Part print with two shaded views. Sizes in mm from the minimum x, y, z corner. Give positions to 0.01 mm unless a question says otherwise; leave off trailing zeros. Order: outer loops, then holes, each group sorted by start corner. A loop starts at its lowest first (then second) coordinate and runs counter-clockwise, first axis right, second up. Notation, with made-up numbers: M 3.25,5 L 27.25,5 A22 cw 27.25,16 Z; hole C 59,-27.75 d6. An arc over 180 degrees is marked long. Write each question's results on one line, items separated by ' | '. Start each with the question number.
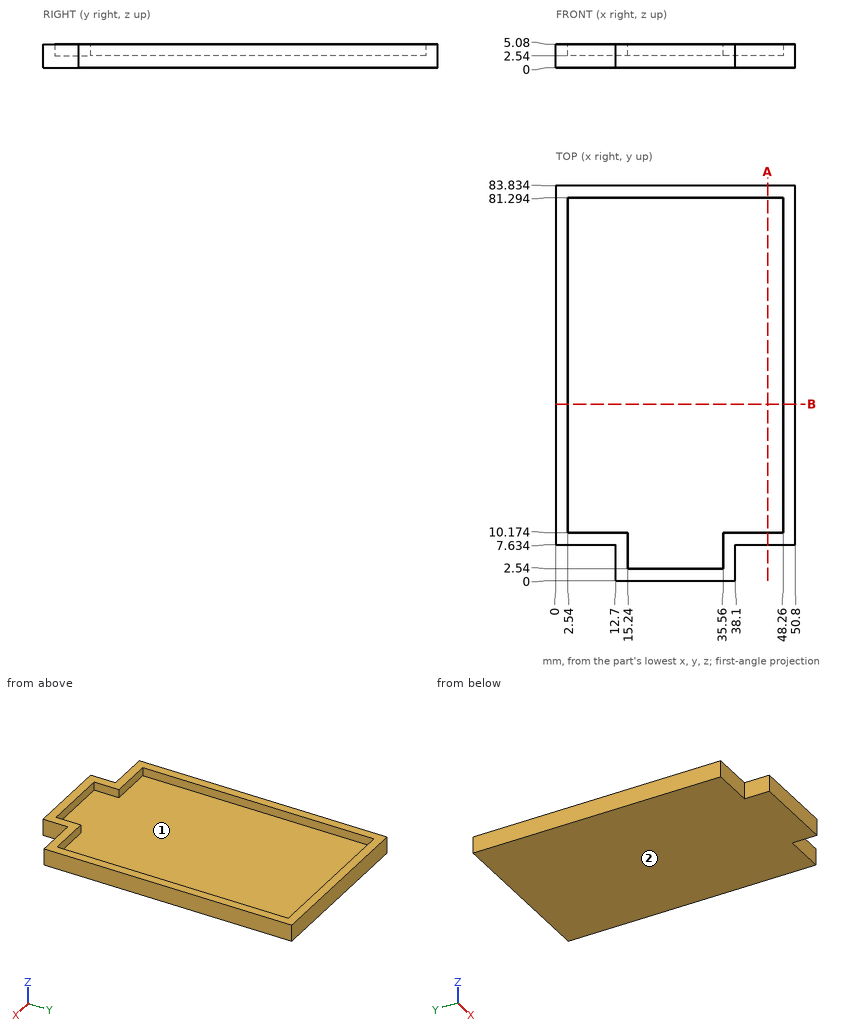
(1) Pull direction Y, two halves, no side cores. Call the marked faces 1 and 2: +Y half, -Y half, draft (parallel to the pull), parting line (faces both ways), or undercut.
(2) Drop flat-ended pins along their axis: P1, Ø4, axis at x = 45.5, y = 31.5, coming from the +Z side; P2, Ø1.3, axis at y = 6.5, z = 3.5, coming from the -X side; P3, Ø2.5, axis at x = 7, z = 1.5, coming from the -Y side. Give the stop position or say it passes through.
(3) Probe L1, parallel to Y at x = 40, z = 4.05; L2, parallel to Y at x = 22, z = 2.7; L3, parallel to X at y = 57, z = 3.05. List the from-to ranges inside material, lowest first.
(4) Saw through at A-A on x = 45. Give the cut face in (y, z).
(5) Saw through at B-B on y = 37.5. Give the cut face in (x, z), plus the area to 3 significant figures.
Taken from the geometry:
1) face 1: undercut | face 2: draft
2) P1: stops at z = 2.54 | P2: stops at x = 12.7 | P3: stops at y = 7.63
3) L1: y = 7.63 to 10.17, 81.29 to 83.83 | L2: y = 0 to 2.54, 81.29 to 83.83 | L3: x = 0 to 2.54, 48.26 to 50.8
4) outline: M 7.63,0 L 83.83,0 L 83.83,5.08 L 81.29,5.08 L 81.29,2.54 L 10.17,2.54 L 10.17,5.08 L 7.63,5.08 Z
5) outline: M 0,0 L 50.8,0 L 50.8,5.08 L 48.26,5.08 L 48.26,2.54 L 2.54,2.54 L 2.54,5.08 L 0,5.08 Z | area: 142 mm²
